Could you check a few things on this model? Use its own coordinates, in mm. Coordinates: 2 decimals unless noted, no trailing zeros. Loops run counter-clockwise (first coordinate to the right, second up) from the corner with the lowest first, then second, coordinate; pieces in that order, holes last.
1) Imagine slicing it at D-D on y = 2.25. Please give me the cut outline in (x, z).
2) Imagine slicing it at A-A on x = 0. Please give me the cut outline in (y, z).
3) Imagine slicing it at C-C on z = -5. Please give me the cut outline in (x, y).
4) Imagine slicing it at B-B on z = 0. Please give me the cut outline in (x, y).
5) If I drill on line 1 along X through (y, z) = (6, 0); line 2 along Z through (x, y) = (7, 4); line 3 along Z through (x, y) = (7.25, 8.5) (3 decimals), over which ranges is the centre line in solid material (lowest first)?
6) Thinking about a two-plate mould opening in Z: for faces 1 (the face through (6.795, 5.063, 4.638)), 2 (the face through (5, 0.526, 3)), 3 (the face through (-2.715, 4.937, 12.228)), which applies, released by +Z, released by -Z, zero draft, split by the parting line, or undercut?
7) Will these pins go through, and if not, where does the flat tip stop? P1, Ø2, axis at x = -6, y = 4, coming from the +Z side; P2, Ø8.5, axis at x = 0, z = 0, coming from the +Y side; P3, Ø3, axis at x = 8.14, z = -4.7, coming from the -Y side; P4, Ø3, axis at x = 4.5, y = 7.5, coming from the +Z side.
```python
from build123d import *

# Parameters (mm, degrees)
SKETCH1_R           = 14
BOSS_EXTRUDE1_DEPTH = 10
SKETCH2_R           = 1.5
SKETCH2_R_2         = 6
CUT_EXTRUDE1_DEPTH  = 11
SCALE_1_SCALE       = 0.894736842


with BuildPart() as part:
    # Sketch1 → Boss-Extrude1 (new body)
    with BuildSketch(Plane(origin=(0, 0, 0), x_dir=(1, 0, 0), z_dir=(0, 1, 0))):
        Circle(SKETCH1_R)
    extrude(amount=BOSS_EXTRUDE1_DEPTH)

    # Sketch2 → Cut-Extrude1 (cut, through all)
    with BuildSketch(Plane(origin=(0, 10, 0), x_dir=(1, 0, 0), z_dir=(0, 1, 0))):
        with Locations((0, 10.5)):
            Circle(SKETCH2_R)
        Circle(SKETCH2_R_2)
        with Locations((9.09326674, 5.25)):
            Circle(SKETCH2_R)
        with Locations((9.09326674, -5.25)):
            Circle(SKETCH2_R)
        with Locations((0, -10.5)):
            Circle(SKETCH2_R)
        with Locations((-9.09326674, -5.25)):
            Circle(SKETCH2_R)
        with Locations((-9.09326674, 5.25)):
            Circle(SKETCH2_R)
    extrude(amount=-CUT_EXTRUDE1_DEPTH, mode=Mode.SUBTRACT)


with BuildPart() as part_1:
    # ｽｹｰﾙ1: scaled about (0, 5, 0)
    add(part.part.scale(SCALE_1_SCALE).moved(Location((0, 0.526315789, 0))))


solid = part_1.part
```
Filled in:
1. outline: circle Ø25.05 at (0, 0); hole circle Ø2.68 at (-8.14, -4.7); hole circle Ø2.68 at (-8.14, 4.7); hole circle Ø10.74 at (0, 0); hole circle Ø2.68 at (0, -9.39); hole circle Ø2.68 at (0, 9.39); hole circle Ø2.68 at (8.14, -4.7); hole circle Ø2.68 at (8.14, 4.7)
2. outline: (0.53, -12.53) - (9.47, -12.53) - (9.47, -10.74) - (0.53, -10.74) - close; (0.53, -8.05) - (9.47, -8.05) - (9.47, -5.37) - (0.53, -5.37) - close; (0.53, 5.37) - (9.47, 5.37) - (9.47, 8.05) - (0.53, 8.05) - close; (0.53, 10.74) - (9.47, 10.74) - (9.47, 12.53) - (0.53, 12.53) - close
3. outline: (-11.49, 0.53) - (-9.44, 0.53) - (-9.44, 9.47) - (-11.49, 9.47) - close; (-6.83, 0.53) - (-1.95, 0.53) - (-1.95, 9.47) - (-6.83, 9.47) - close; (1.95, 0.53) - (6.83, 0.53) - (6.83, 9.47) - (1.95, 9.47) - close; (9.44, 0.53) - (11.49, 0.53) - (11.49, 9.47) - (9.44, 9.47) - close
4. outline: (-12.53, 0.53) - (-5.37, 0.53) - (-5.37, 9.47) - (-12.53, 9.47) - close; (5.37, 0.53) - (12.53, 0.53) - (12.53, 9.47) - (5.37, 9.47) - close
5. line 1: x = -12.53 to -5.37, 5.37 to 12.53
5. line 2: z = -10.39 to -5.41, -3.98 to 3.98, 5.41 to 10.39
5. line 3: z = -10.215 to -5.705, -3.689 to 3.689, 5.705 to 10.215
6. face 1: undercut
6. face 2: zero draft
6. face 3: split by the parting line
7. P1: stops at z = 11.49
7. P2: passes through
7. P3: stops at y = 0.53
7. P4: stops at z = 12.16
